Can you work these out from the model? Positions are in its coordinate system, mm. Face numbers are marked on the shaded views. A direction names the side the tool comes from. Round coordinates to 2 decimals unless told otherwise and drop trailing zeros. Order: outer loops, then holes, each group sorted by start corner. A loop starts at its lowest first (then second) coordinate and runs counter-clockwise, first axis right, second up.
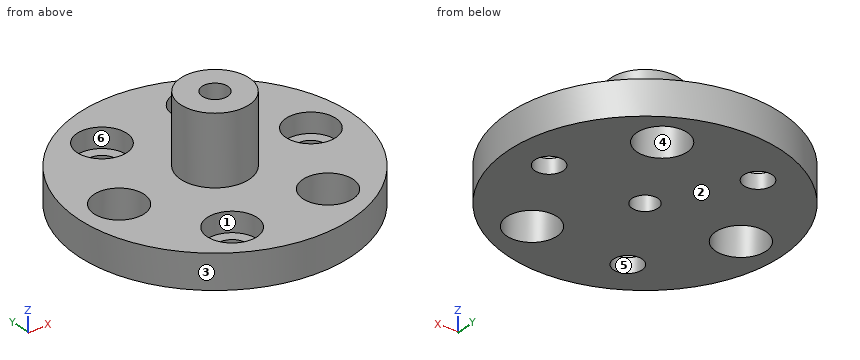
from build123d import *

# Parameters (mm, degrees)
CROQUIS1_R              = 15.9
CROQUIS1_R_2            = 2.925
CROQUIS1_R_3            = 1.65
CROQUIS1_R_4            = 1.5
SALIENTE_EXTRUIR1_DEPTH = 4
CROQUIS3_R              = 4
CROQUIS3_R_2            = 1.5
SALIENTE_EXTRUIR3_DEPTH = 8
CROQUIS4_R              = 2.9
CORTAR_EXTRUIR2_DEPTH   = 2.3


with BuildPart() as part:
    # Croquis1 → Saliente-Extruir1 (new body)
    with BuildSketch(Plane.XY.offset(998.15499802)):
        with Locations((2.956072514, 15.206748875)):
            Circle(CROQUIS1_R)
        with Locations((-8.293927486, 15.206748875)):
            Circle(CROQUIS1_R_2, mode=Mode.SUBTRACT)
        with Locations((14.206072514, 15.206748875)):
            Circle(CROQUIS1_R_3, mode=Mode.SUBTRACT)
        with Locations((-2.668927486, 5.463963082)):
            Circle(CROQUIS1_R_3, mode=Mode.SUBTRACT)
        with Locations((-2.668927486, 24.949534667)):
            Circle(CROQUIS1_R_3, mode=Mode.SUBTRACT)
        with Locations((8.581072514, 24.949534667)):
            Circle(CROQUIS1_R_2, mode=Mode.SUBTRACT)
        with Locations((2.956072514, 15.206748875)):
            Circle(CROQUIS1_R_4, mode=Mode.SUBTRACT)
        with Locations((8.581072514, 5.463963082)):
            Circle(CROQUIS1_R_2, mode=Mode.SUBTRACT)
    extrude(amount=SALIENTE_EXTRUIR1_DEPTH)

    # Croquis3 → Saliente-Extruir3 (add)
    with BuildSketch(Plane.XY.offset(1002.15499802)):
        with Locations((2.956072514, 15.206748875)):
            Circle(CROQUIS3_R)
        with Locations((2.956072514, 15.206748875)):
            Circle(CROQUIS3_R_2, mode=Mode.SUBTRACT)
    extrude(amount=SALIENTE_EXTRUIR3_DEPTH)

    # Croquis4 → Cortar-Extruir2 (cut)
    with BuildSketch(Plane.XY.offset(1002.15499802)):
        with Locations((-2.668927486, 24.949534667)):
            Circle(CROQUIS4_R)
        with Locations((14.206072514, 15.206748875)):
            Circle(CROQUIS4_R)
        with Locations((-2.668927486, 5.463963082)):
            Circle(CROQUIS4_R)
    extrude(amount=-CORTAR_EXTRUIR2_DEPTH, mode=Mode.SUBTRACT)


solid = part.part
(1) On a 3-axis mill with a long thin cutter (end or side, diameter ignored), from which of +Z, -Z, +X, -X, +Y, -Y can I reach the whole of each face in a straight line? I mean the marked faces 5 and 6. Say none if no direction works.
(2) If we mould it in two halves opening along Y, with no side actions, what happens to the marked faces 1, 2, 3 and 4? For each: pulls with the +Y half, pulls with the -Y half, needs draft (parallel to the pull), parting line crosses it, or undercut.
(3) I want a section at C-C, the plane z = 1001.75. List the corners of the cut face in (x, y) for me (3 decimals), plus the area to 3 significant figures.
(4) I want a section at A-A, the plane y = 27. List the corners of the cut face in (x, z) for me (3 decimals).
(5) Please list where these lines run through material, in increasing order: probe 1 along Y at (x, z) = (3, 1005); probe 2 along X at (y, z) = (14, 1008.75); probe 3 along Z at (x, y) = (14, 7) (3 decimals).
(6) I want a section at B-B, the plane x = 10.5. List the corners of the cut face in (y, z) for me (3 decimals), plus the area to 4 significant figures.
(7) I want a section at D-D, the plane y = 6. List the corners of the cut face in (x, z) for me (3 decimals).
(8) I'm going to push flat-ended pins straight in: pin 1 Ø5.5 at (x, y) = (-2.67, 5.46) entering from +Z (3 decimals); pin 2 Ø3 at (x, y) = (14.21, 15.21) entering from +Z; pin 3 Ø6 at (y, z) = (18.5, 1000) entering from +X; pin 4 Ø6 at (x, z) = (-3.5, 1007.5) entering from +Y. Where does each tip first touch, or does it pass through?
Ans:
1. face 5: +Z, -Z
1. face 6: +Z
2. face 1: undercut
2. face 2: needs draft
2. face 3: parting line crosses it
2. face 4: undercut
3. outline: circle Ø31.8 at (2.956, 15.207); hole circle Ø5.85 at (-8.294, 15.207); hole circle Ø5.8 at (-2.669, 5.464); hole circle Ø5.8 at (-2.669, 24.95); hole circle Ø3 at (2.956, 15.207); hole circle Ø5.85 at (8.581, 5.464); hole circle Ø5.85 at (8.581, 24.95); hole circle Ø5.8 at (14.206, 15.207)
3. area: 627 mm2
4. outline: (-7.708, 998.155) - (6.495, 998.155) - (6.495, 1002.155) - (-0.618, 1002.155) - (-0.618, 999.855) - (-4.72, 999.855) - (-4.72, 1002.155) - (-7.708, 1002.155) - close; (10.667, 998.155) - (13.62, 998.155) - (13.62, 1002.155) - (10.667, 1002.155) - close
5. probe 1: y = 11.21 to 13.71, 16.71 to 19.21
5. probe 2: x = -0.86 to 2.07, 3.85 to 6.77
5. probe 3: z = 998.155 to 1002.155
6. outline: (1.21, 998.155) - (3.256, 998.155) - (3.256, 1002.155) - (1.21, 1002.155) - close; (7.672, 998.155) - (22.742, 998.155) - (22.742, 1002.155) - (7.672, 1002.155) - close; (27.157, 998.155) - (29.203, 998.155) - (29.203, 1002.155) - (27.157, 1002.155) - close
6. area: 76.65 mm2
7. outline: (-10.007, 998.155) - (-4.229, 998.155) - (-4.229, 999.855) - (-5.519, 999.855) - (-5.519, 1002.155) - (-10.007, 1002.155) - close; (-1.108, 998.155) - (5.706, 998.155) - (5.706, 1002.155) - (0.181, 1002.155) - (0.181, 999.855) - (-1.108, 999.855) - close; (11.457, 998.155) - (15.919, 998.155) - (15.919, 1002.155) - (11.457, 1002.155) - close
8. pin 1: stops at z = 999.855
8. pin 2: passes through
8. pin 3: stops at x = 18.85
8. pin 4: stops at y = 17.22
